The model under review builds one solid part; all positions refer to its coordinate system, in mm. A direction names the side the tool comes from. Round coordinates to 2 decimals unless told otherwise and drop trailing zeros. Write each loop counter-clockwise with the first axis right and the second up, starting at its lowest first coordinate (ties: lowest second). Pieces come first, ordered by that corner, then holes.
Item 1: Add section D-D (z = -11). Give the boundary of the cut face in (x, y) (3 decimals).
Item 2: Draft analysis for pull direction X (two halves, no side actions). For faces 4 (the face through (-21, 5.665, -43)), 5 (the face through (14, -1, 20)), 6 (the face through (59.82, 0.08, 43)), state which applies: +X half, -X half, draft (parallel to the pull), parting line (faces both ways), or undercut.
Item 3: Clearance check with flat-ended pins moving along their axes: pin 1 Ø1 at (x, z) = (-55.5, -37) entering from +Y (3 decimals); pin 2 Ø2 at (x, z) = (-60, -4) entering from +Y (3 decimals); pin 3 Ø4 at (x, z) = (40, -4) entering from +Y (3 decimals). State where each tip first meets the part, or that it passes through.
Item 4: Add section C-C (x = 45.5). Give the boundary of the cut face in (y, z) (3 decimals), plus the area to 3 significant figures.
Item 5: Add section B-B (x = -11). Give the boundary of the cut face in (y, z) (3 decimals), plus the area to 3 significant figures.
Item 6: Machinability: for faces 1 (the face through (31, 5.665, 43)), 2 (the face through (40, -4.665, 1)), 3 (the face through (58.39, 0.93, 41.6)), which of the approach directions +Z, -Z, +X, -X, +Y, -Y give a long, thin tool a straight path to every point of the face, cutting with its end or side? Answer none if there is none.
Item 7: Add section A-A (z = -30.5). Give the boundary of the cut face in (x, y) (3 decimals).
Item 8: To check wall thickness, follow L1, parallel to X at y = -0.35, z = -36.46; L2, parallel to X at y = -3.5, z = -8; L3, parallel to X at y = -5.4, z = -4. State the ranges of each line that lie inside material, in increasing order.
```python
from build123d import *
from OCP.BRepFilletAPI import BRepFilletAPI_MakeFillet

# Parameters (mm, degrees)
SKETCH1_W           = 122.5
SKETCH1_H           = 89
BOSS_EXTRUDE1_DEPTH = 5.665
SHELL1_T            = -2
SKETCH2_R           = 2.5
SKETCH2_R_2         = 1
BOSS_EXTRUDE2_DEPTH = 6
FILLET1_R1          = 3
FILLET1_R2          = 5
SKETCH6_W           = 2
SKETCH6_H           = 66
CUT_EXTRUDE1_DEPTH  = 2.4
SKETCH7_W           = 2
SKETCH7_H           = 17.347336969
CUT_EXTRUDE2_DEPTH  = 8.57
CUT_EXTRUDE5_DEPTH  = 10
SKETCH13_W          = 32.782947734
SKETCH13_H          = 2.623502387
CUT_EXTRUDE6_DEPTH  = 10
SKETCH14_W          = 54
SKETCH14_H          = 44
SKETCH14_W_2        = 50
SKETCH14_H_2        = 40
BOSS_EXTRUDE3_DEPTH = 5
SKETCH15_W          = 2
SKETCH15_H          = 4
SKETCH15_W_2        = 4
SKETCH15_H_2        = 2
CUT_EXTRUDE7_DEPTH  = 5
CUT_EXTRUDE9_DEPTH  = 1
SKETCH17_R          = 1
CUT_EXTRUDE10_DEPTH = 1


with BuildPart() as part:
    # Sketch1 → Boss-Extrude1 (new, symmetric)
    with BuildSketch(Plane(origin=(0, 0, 0), x_dir=(1, 0, 0), z_dir=(0, 1, 0))):
        Rectangle(SKETCH1_W, SKETCH1_H)
    extrude(amount=BOSS_EXTRUDE1_DEPTH, both=True)

    # Shell1
    shell1_openings = [part.faces().sort_by_distance(p)[0] for p in [
        (0, 5.665, 0),
    ]]
    offset(amount=SHELL1_T, openings=shell1_openings, kind=Kind.INTERSECTION)

    # Sketch2 → Boss-Extrude2 (add)
    # profile 1 of 3: a face of its own
    with BuildSketch(Plane(origin=(0, -3.665, 0), x_dir=(1, 0, 0), z_dir=(0, 1, 0))):
        with Locations(Location((-55.52, 36.46, 0), (0, 0, 270))):
            Circle(SKETCH2_R)
        with Locations(Location((-55.52, 36.46, 0), (0, 0, 270))):
            Circle(SKETCH2_R_2, mode=Mode.SUBTRACT)
    # profile 2 of 3: a face of its own
    with BuildSketch(Plane(origin=(0, -3.665, 0), x_dir=(1, 0, 0), z_dir=(0, 1, 0))):
        with Locations(Location((51.52, 36.46, 0), (0, 0, 270))):
            Circle(SKETCH2_R)
        with Locations(Location((51.52, 36.46, 0), (0, 0, 270))):
            Circle(SKETCH2_R_2, mode=Mode.SUBTRACT)
    # profile 3 of 3: a face of its own
    with BuildSketch(Plane(origin=(0, -3.665, 0), x_dir=(1, 0, 0), z_dir=(0, 1, 0))):
        with Locations(Location((-55.52, -36.46, 0), (0, 0, 270))):
            Circle(SKETCH2_R)
        with Locations(Location((-55.52, -36.46, 0), (0, 0, 270))):
            Circle(SKETCH2_R_2, mode=Mode.SUBTRACT)
    extrude(amount=BOSS_EXTRUDE2_DEPTH)

    # Fillet1: one fillet with a radius per group of edges: ONE call of the kernel's fillet builder (fillet() takes one radius for all edges)
    fillet1_edges_1 = [part.edges().sort_by_distance(p)[0] for p in [
        (-59.25, 1, -42.5),
        (59.25, 1, -42.5),
        (59.25, 1, 42.5),
        (-59.25, 1, 42.5),
    ]]
    fillet1_edges_2 = [part.edges().sort_by_distance(p)[0] for p in [
        (-61.25, 0, -44.5),
        (61.25, 0, -44.5),
        (61.25, 0, 44.5),
        (-61.25, 0, 44.5),
    ]]
    fillet1 = BRepFilletAPI_MakeFillet(part.part.solid().wrapped)
    for e in fillet1_edges_1:
        fillet1.Add(FILLET1_R1, e.wrapped)
    for e in fillet1_edges_2:
        fillet1.Add(FILLET1_R2, e.wrapped)
    add(Compound.cast(fillet1.Shape()), mode=Mode.REPLACE)

    # Sketch6 → Cut-Extrude1 (cut)
    with BuildSketch(Plane(origin=(0, 5.665, 0), x_dir=(1, 0, 0), z_dir=(0, 1, 0))):
        with Locations((-60.25, 0)):
            Rectangle(SKETCH6_W, SKETCH6_H)
    extrude(amount=-CUT_EXTRUDE1_DEPTH, mode=Mode.SUBTRACT)

    # Sketch7 → Cut-Extrude2 (cut)
    with BuildSketch(Plane(origin=(0, 5.665, 0), x_dir=(1, 0, 0), z_dir=(0, 1, 0))):
        with Locations((60.25, -29.826331516)):
            Rectangle(SKETCH7_W, SKETCH7_H)
    extrude(amount=-CUT_EXTRUDE2_DEPTH, mode=Mode.SUBTRACT)

    # Sketch12 → Cut-Extrude5 (cut)
    with BuildSketch(Plane(origin=(0, 0, -44.5), x_dir=(-1, 0, 0), z_dir=(0, 0, -1))):
        with BuildLine():
            Line((-42.852887486, 5.665199886), (-33.912887486, 5.665199886))
            Line((-33.912887486, 5.665199886), (-33.612887486, 5.665))
            Line((-33.612887486, 5.665), (-33.612887486, 5.335199886))
            add(Edge.make_bspline(
                [(-35.162887486, 3.785199886), (-34.969276417, 3.785199886), (-34.590674628, 3.851796456), (-34.032768291, 4.205080692), (-33.679484056, 4.762987029), (-33.612887486, 5.141588818), (-33.612887486, 5.335199886)],
                knots=[0, 0, 0, 0, 0.25, 0.5, 0.75, 1, 1, 1, 1], degree=3))
            Line((-35.162887486, 3.785199886), (-41.602887486, 3.785199886))
            add(Edge.make_bspline(
                [(-43.152887486, 5.335199886), (-43.152887486, 5.141588818), (-43.086290916, 4.762987029), (-42.73300668, 4.205080692), (-42.175100343, 3.851796456), (-41.796498554, 3.785199886), (-41.602887486, 3.785199886)],
                knots=[0, 0, 0, 0, 0.25, 0.5, 0.75, 1, 1, 1, 1], degree=3))
            Line((-43.152887486, 5.335199886), (-43.152887486, 5.665))
            Line((-43.152887486, 5.665), (-42.852887486, 5.665199886))
        make_face()
    extrude(amount=-CUT_EXTRUDE5_DEPTH, mode=Mode.SUBTRACT)

    # Sketch13 → Cut-Extrude6 (cut)
    with BuildSketch(Plane.XY.offset(44.5)):
        with Locations((-20.613592251, 5.246951194)):
            Rectangle(SKETCH13_W, SKETCH13_H)
    extrude(amount=-CUT_EXTRUDE6_DEPTH, mode=Mode.SUBTRACT)

    # Sketch14 → Boss-Extrude3 (add)
    with BuildSketch(Plane(origin=(0, -3.665, 0), x_dir=(1, 0, 0), z_dir=(0, 1, 0))):
        Rectangle(SKETCH14_W, SKETCH14_H)
        Rectangle(SKETCH14_W_2, SKETCH14_H_2, mode=Mode.SUBTRACT)
    extrude(amount=BOSS_EXTRUDE3_DEPTH)

    # Sketch15 → Cut-Extrude7 (cut)
    with BuildSketch(Plane(origin=(0, 1.335, 0), x_dir=(1, 0, 0), z_dir=(0, 1, 0))):
        with Locations((-26, 18)):
            Rectangle(SKETCH15_W, SKETCH15_H)
        with Locations((-26, 0)):
            Rectangle(SKETCH15_W, SKETCH15_H)
        with Locations((-26, -18)):
            Rectangle(SKETCH15_W, SKETCH15_H)
        with Locations((26, -18)):
            Rectangle(SKETCH15_W, SKETCH15_H)
        with Locations((26, 0)):
            Rectangle(SKETCH15_W, SKETCH15_H)
        with Locations((26, 18)):
            Rectangle(SKETCH15_W, SKETCH15_H)
        with Locations((0, 21)):
            Rectangle(SKETCH15_W_2, SKETCH15_H_2)
        with Locations((0, -21)):
            Rectangle(SKETCH15_W_2, SKETCH15_H_2)
    extrude(amount=-CUT_EXTRUDE7_DEPTH, mode=Mode.SUBTRACT)

    # Sketch16 → Cut-Extrude9 (cut)
    with BuildSketch(Plane.XZ.offset(5.665)):
        with BuildLine():
            ThreePointArc((37.917995747, -2.616071429), (40, -6.5), (42.082004253, -2.616071429))
            ThreePointArc((42.082004253, -2.616071429), (41.931122098, -1.882594271), (42.331844763, -1.25))
            ThreePointArc((42.331844763, -1.25), (40, 6), (37.668155237, -1.25))
            ThreePointArc((37.668155237, -1.25), (38.068877902, -1.882594271), (37.917995747, -2.616071429))
        make_face()
        with BuildLine():
            ThreePointArc((-42.082004253, -2.616071429), (-40, -6.5), (-37.917995747, -2.616071429))
            ThreePointArc((-37.917995747, -2.616071429), (-38.068877902, -1.882594271), (-37.668155237, -1.25))
            ThreePointArc((-37.668155237, -1.25), (-40, 6), (-42.331844763, -1.25))
            ThreePointArc((-42.331844763, -1.25), (-41.931122098, -1.882594271), (-42.082004253, -2.616071429))
        make_face()
    extrude(amount=-CUT_EXTRUDE9_DEPTH, mode=Mode.SUBTRACT)

    # Sketch17 → Cut-Extrude10 (cut)
    with BuildSketch(Plane.XZ.offset(4.665)):
        with Locations(Location((-40, -4, 0), (0, 0, 270))):
            Circle(SKETCH17_R)
        with Locations(Location((40, -4, 0), (0, 0, 270))):
            Circle(SKETCH17_R)
    extrude(amount=-CUT_EXTRUDE10_DEPTH, mode=Mode.SUBTRACT)


solid = part.part
```
Numbers:
1. outline: (-61.25, -5.665) - (61.25, -5.665) - (61.25, 5.665) - (59.25, 5.665) - (59.25, -3.665) - (27, -3.665) - (27, 1.335) - (25, 1.335) - (25, -3.665) - (-25, -3.665) - (-25, 1.335) - (-27, 1.335) - (-27, -3.665) - (-59.25, -3.665) - (-59.25, 3.265) - (-61.25, 3.265) - close
2. face 4: draft
2. face 5: undercut
2. face 6: +X half
3. pin 1: stops at y = 2.335
3. pin 2: stops at y = 3.265
3. pin 3: stops at y = -3.665
4. outline: (-5.665, -44.5) - (5.665, -44.5) - (5.665, -42.5) - (-3.665, -42.5) - (-3.665, 42.5) - (5.665, 42.5) - (5.665, 44.5) - (-5.665, 44.5) - close
4. area: 215 mm2
5. outline: (-5.665, -44.5) - (5.665, -44.5) - (5.665, -42.5) - (-3.665, -42.5) - (-3.665, -22) - (1.335, -22) - (1.335, -20) - (-3.665, -20) - (-3.665, 20) - (1.335, 20) - (1.335, 22) - (-3.665, 22) - (-3.665, 42.5) - (3.935, 42.5) - (3.935, 44.5) - (-5.665, 44.5) - close
5. area: 232 mm2
6. face 1: +Z, -Z, +X, -X, +Y
6. face 2: -Y
6. face 3: +Y
7. outline: (-61.25, -5.665) - (61.25, -5.665) - (61.25, 5.665) - (59.25, 5.665) - (59.25, -3.665) - (-59.25, -3.665) - (-59.25, 3.265) - (-61.25, 3.265) - close
8. L1: x = -61.25 to -59.25, -58.02 to -56.52, -54.52 to -53.02, 49.02 to 50.52, 52.52 to 54.02, 59.25 to 61.25
8. L2: x = -61.25 to -59.25, -27 to -25, 25 to 27, 59.25 to 61.25
8. L3: x = -61.25 to -42.5, -37.5 to 37.5, 42.5 to 61.25
